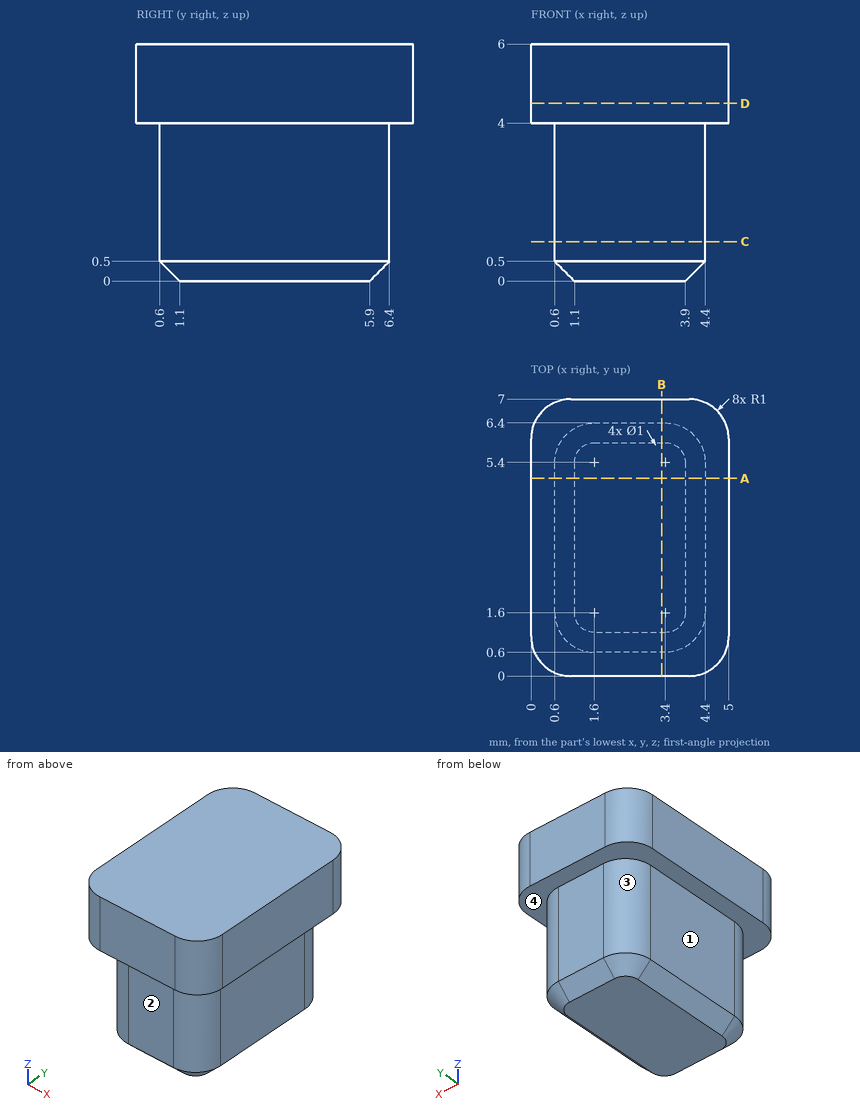
Answer from the drawing. Dimensions are ordinates in mm from the lowest x, y and z of the part. A direction names the side the tool comes from. Round coordinates to 2 decimals unless told otherwise and drop trailing zeros. Loops run counter-clockwise (first coordinate to the right, second up) from the corner with the lowest first, then second, coordinate; pieces in that order, holes last.
Q1. Consider probe 1 along Y at (x, z) = (3, 3.7); probe 2 along X at (y, z) = (3, 1.65); probe 3 along Z at (x, y) = (0.55, 5.5). Determine where each line is inside the solid, lowest interval first.
Q2. Which of the six approach directions +Z, -Z, +X, -X, +Y, -Y give full straight-line access (tool end or side, diameter ignored) to the marked faces 1, 2, 3 and 4?
Q3. Section A-A on y = 5 is taken. Write down the section's boundary in (x, z), and give its area (4 significant figures).
Q4. Section D-D on z = 4.5 is taken. Write down the section's boundary in (x, y), and give its area (3 significant figures).
Q5. Section B-B on x = 3.3 is taken. Write down the section's boundary in (y, z).
Q6. Section C-C on z = 1 is taken. Write down the section's boundary in (x, y).
Q7. Each of these flat-tipped pins is pushed along its axis until it touches: pin 1 (1 mm diameter, centred on x = 4.5, z = 3, fed in from +Y); pin 2 (3 mm diameter, centred on y = 3.5, z = 2, fed in from +X); pin 3 (2 mm diameter, centred on x = 2, z = 2.5, fed in from +Y). Where does it stop, or does it pass through?
Output:
1. probe 1: y = 0.6 to 6.4
1. probe 2: x = 0.6 to 4.4
1. probe 3: z = 4 to 6
2. face 1: -Z, -X, +Y, -Y
2. face 2: -Z, +X, -X, -Y
2. face 3: -Z, -X, +Y
2. face 4: -Z
3. outline: (0, 4) - (0.6, 4) - (0.6, 0.5) - (1.1, 0) - (3.9, 0) - (4.4, 0.5) - (4.4, 4) - (5, 4) - (5, 6) - (0, 6) - close
3. area: 24.95 mm2
4. outline: (0, 1) arc R1 ccw to (1, 0) - (4, 0) arc R1 ccw to (5, 1) - (5, 6) arc R1 ccw to (4, 7) - (1, 7) arc R1 ccw to (0, 6) - close
4. area: 34.1 mm2
5. outline: (0, 4) - (0.6, 4) - (0.6, 0.5) - (1.1, 0) - (5.9, 0) - (6.4, 0.5) - (6.4, 4) - (7, 4) - (7, 6) - (0, 6) - close
6. outline: (0.6, 1.6) arc R1 ccw to (1.6, 0.6) - (3.4, 0.6) arc R1 ccw to (4.4, 1.6) - (4.4, 5.4) arc R1 ccw to (3.4, 6.4) - (1.6, 6.4) arc R1 ccw to (0.6, 5.4) - close
7. pin 1: stops at y = 6.2
7. pin 2: stops at x = 4.4
7. pin 3: stops at y = 6.4
